Could you check a few things on this model? Use its own coordinates, in mm. A direction names the side the tool comes from. Coordinates: 2 decimals unless noted, no trailing zeros. Loops run counter-clockwise (first coordinate to the right, second up) from the corner with the lowest first, then second, coordinate; pieces in that order, holes last. Notation, with made-up numbers: M 4.25,-20.5 L 9.25,-20.5 A10 cw 9.25,-7.5 Z; hole C 65.5,21.5 d2. An arc over 180 degrees is marked long. Return JSON: item names as keys, results as strings. Group by question number.
Autodesk Inventor part; units mm, degrees
ref_plane "Płaszczyzna konstrukcyjna1" through (-7.9876, -5.0569, -14.5) normal (0, -1, 0) x (1, 0, 0)
ref_plane "YZ Plane" through (0, 0, 0) normal (1, 0, 0) x (0, 1, 0)
ref_plane "XZ Plane" through (0, 0, 0) normal (0, 1, 0) x (-1, 0, 0)
sketch "Szkic1" plane through (0, 0, 0) normal (0, 0, 1) x (1, 0, 0)
  line L0 (-6.6876, 6.2431) -> (12.1124, 6.2431)
  line L1 (12.1124, 6.2431) -> (12.1124, -6.2569)
  line L2 (12.1124, -6.2569) -> (-6.6876, -6.2569)
  line L3 (-6.6876, -6.2569) -> (-6.6876, 6.2431)
  line L4 (-3.9802, 2.2431) -> (-3.2802, 2.2431)
  line L5 (-3.2802, 2.2431) -> (-3.2802, -2.2569)
  line L6 (-3.2802, -2.2569) -> (-3.9802, -2.2569)
  line L7 (-3.9802, -2.2569) -> (-3.9802, 2.2431)
  line L8 (2.3508, 2.2431) -> (3.0508, 2.2431)
  line L9 (3.0508, 2.2431) -> (3.0508, -2.2569)
  line L10 (3.0508, -2.2569) -> (2.3508, -2.2569)
  line L11 (2.3508, -2.2569) -> (2.3508, 2.2431)
  line L12 (9.1799, 2.2431) -> (9.8799, 2.2431)
  line L13 (9.8799, 2.2431) -> (9.8799, -2.2569)
  line L14 (9.8799, -2.2569) -> (9.1799, -2.2569)
  line L15 (9.1799, -2.2569) -> (9.1799, 2.2431)
  point P0 (0, 0)
  dimension "d0" = 18.8
  dimension "d1" = 12.5
  dimension "d2" = 0.7
  dimension "d3" = 4.5
  dimension "d4" = 4
  dimension "d5" = 0.7
  dimension "d6" = 4.5
  dimension "d7" = 0.7
  dimension "d8" = 4.5
extrude "Wyciągnięcie proste1" add sketch "Szkic1" against normal blind 14.5 contours L0 L1 L2 L3 | L4 L5 L6 L7 | L8 L9 L10 L11 | L12 L13 L14 L15
extrude "Wyciągnięcie proste2" add sketch "Szkic1" along normal blind 8 contours L4 L5 L6 L7 | L8 L9 L10 L11 | L12 L13 L14 L15
fillet "Zaokrąglenie1" radius 1.5 6 edges at (-3.6302, 2.2431, 8) (2.7008, 2.2431, 8) (9.5299, 2.2431, 8) (-3.6302, -2.2569, 8) (2.7008, -2.2569, 8) (9.5299, -2.2569, 8)
sketch "Szkic2" plane through (0, 0, -14.5) normal (0, 0, -1) x (-1, 0, 0)
  line L0 (6.6876, 6.2431) -> (-12.1124, 6.2431)
  line L1 (-12.1124, 6.2431) -> (-12.1124, -6.2569)
  line L2 (-12.1124, -6.2569) -> (6.6876, -6.2569)
  line L3 (6.6876, -6.2569) -> (6.6876, 6.2431)
  line L4 (-13.4124, 7.5431) -> (7.9876, 7.5431)
  line L5 (7.9876, 7.5431) -> (7.9876, -7.5569)
  line L6 (7.9876, -7.5569) -> (-13.4124, -7.5569)
  line L7 (-13.4124, -7.5569) -> (-13.4124, 7.5431)
  point P0 (0, 0)
  dimension "d14" = 18.8
  dimension "d15" = 1.3
extrude "Wyciągnięcie proste3" add sketch "Szkic2" along normal blind 2 contours L3 L2 L1 L0 | L4 L5 L6 L7
sketch "Szkic3" plane through (-3.9802, -2.2569, 0) normal (-1, 0, 0) x (0, 0, 1)
  line L0 (0, 4.5) -> (6.5, 4.5)
  line L1 (0, 0) -> (6.5, 0)
  point P0 (0, 2.2569)
  point P1 (5.956, 2.25)
  dimension "d18" = 4.5
  dimension "d19" = 2.25
hole "Otwór1" at (-3.9802, -0.0069, 5.956) direction (1, 0, 0) diameter 2 end through all
ref_plane "Płaszczyzna konstrukcyjna1" through (-7.9876, -5.0569, -14.5) normal (0, -1, 0) x (1, 0, 0)
sketch "Szkic4" plane through (-7.9876, -5.0569, -14.5) normal (0, -1, 0) x (1, 0, 0)
  line L0 (21.4, 0) -> (0, 0)
  line L1 (21.4, 0) -> (21.4, -2)
  line L2 (0, -2) -> (21.4, -2)
  line L3 (0, 0) -> (0, -2)
  line L4 (0, -2) -> (21.4, -2)
  arc A0 (15.4, -6) -> (18.4, -2) centre (11.6248, -0.0436) ccw
  line L5 (15.4, -6) -> (2.5, -2)
  point P0 (7.9876, 14.5)
  dimension "d28" = 3
  dimension "d29" = 2.5
  dimension "d30" = 4
  dimension "d31" = 6
extrude "Wyciągnięcie proste4" add sketch "Szkic4" against normal blind 10.1 contours A0 L5 L2
sketch "Szkic5" plane through (-5.4876, -5.0569, -16.5) normal (-0.2962, 0, -0.9551) x (-0.9551, 0, 0.2962)
  line L0 (-13.2267, 2.4266) -> (-13.2267, 8.6477) construction
  line L1 (-13.2267, 8.6477) -> (-8.9095, 8.6477) construction
  line L2 (-8.9095, 8.6477) -> (-8.9095, 2.4266) construction
  line L3 (-8.9095, 2.4266) -> (-13.2267, 2.4266) construction
  line L4 (-6.957, 3.6505) -> (-6.957, 6.2802) construction
  line L5 (-6.957, 6.2802) -> (-0.4173, 6.2802) construction
  line L6 (-0.4173, 6.2802) -> (-0.4173, 3.6505) construction
  line L7 (-0.4173, 3.6505) -> (-6.957, 3.6505) construction
equation "\"d4\" = -0.5 * d3 + 0.5 * d1"
properties part number "COTS_GENERIC_AC_Power_Switch_5A"
(1) For faces 5 (the face through (12.112, 0, -7)), 6 (the face through (3, 7, -14.5)), 7 (the face through (3, 6.243, -7)), 8 (the face through (-6.688, 0, -7)), which set-ups out of +Z, -Z, +X, -X, +Y, -Y let a thin tool reach every point of the face, with its end or its side?
(2) If I drill on L1, parallel to Z at x = 12.5, y = -2.5; L2, parallel to X at y = -3, z = -8; L3, parallel to Y at x = 1.5, z = -1.5, over which ranges is the centre line in solid material (lowest first)? Write a range as [from, to].
(3) Imagine slicing it at D-D, the plane y = 1.5. Write out the boundary of the cut face in (x, z).
(4) We'd pull the mould along X, two halves only. Please class faces 1 (the face through (2.351, 0, 4)), 2 (the face through (9.88, 0, 4)), 3 (the face through (2.706, 1.815, 7.549)), 4 (the face through (9.18, 0, 4)): +X half, -X half, draft (parallel to the pull), parting line (faces both ways), or undercut.
(5) Will these pins go through, and if not, where does the flat tip stop? P1, Ø8, axis at x = 5.5, y = 4, coming from the +Z side; P2, Ø2, axis at x = 0.5, z = -18, coming from the -Y side; P3, Ø12, axis at x = -3, z = 2.5, coming from the +Y side.
(6) Imagine slicing it at A-A, the plane y = 3.5. Write out the boundary of the cut face in (x, z), then the cut area to 3 significant figures.
(7) Imagine slicing it at B-B, the plane x = 7. Write out the boundary of the cut face in (y, z), then the cut area to 3 significant figures.
(8) Imagine slicing it at C-C, the plane z = -18.5. Write out the boundary of the cut face in (x, y).
Checks:
{
 "1": {"face 5": "+Z, +X, +Y, -Y", "face 6": "+Z", "face 7": "+Z, +X, -X, +Y", "face 8": "+Z, -X, +Y, -Y"},
 "2": {"L1": "[-16.5, -14.5]", "L2": "[-6.69, 12.11]", "L3": "[-6.26, 6.24]"},
 "3": {"outline": "M -7.99,-16.5 L -5.49,-16.5 L 7.41,-20.5 A7.05 ccw 10.41,-16.5 L 13.41,-16.5 L 13.41,-14.5 L 12.11,-14.5 L 12.11,0 L 9.88,0 L 9.88,7.8 L 9.18,7.8 L 9.18,0 L 3.05,0 L 3.05,7.8 L 2.35,7.8 L 2.35,0 L -3.28,0 L -3.28,7.8 L -3.98,7.8 L -3.98,0 L -6.69,0 L -6.69,-14.5 L -7.99,-14.5 Z"},
 "4": {"face 1": "undercut", "face 2": "+X half", "face 3": "draft", "face 4": "undercut"},
 "5": {"P1": "z = 8", "P2": "y = -5.06", "P3": "y = 6.24"},
 "6": {"outline": "M -7.99,-16.5 L -5.49,-16.5 L 7.41,-20.5 A7.05 ccw 10.41,-16.5 L 13.41,-16.5 L 13.41,-14.5 L 12.11,-14.5 L 12.11,0 L -6.69,0 L -6.69,-14.5 L -7.99,-14.5 Z", "area": "349 mm²"},
 "7": {"outline": "M -7.56,-16.5 L -5.06,-16.5 L -5.06,-20.37 L 5.04,-20.37 L 5.04,-16.5 L 7.54,-16.5 L 7.54,-14.5 L 6.24,-14.5 L 6.24,0 L -6.26,0 L -6.26,-14.5 L -7.56,-14.5 Z", "area": "251 mm²"},
 "8": {"outline": "M 0.96,-5.06 L 9.47,-5.06 L 9.47,5.04 L 0.96,5.04 Z"}
}
